```python
from build123d import *

# Parameters (mm, degrees)
F0_W     = 2.479451
F0_H     = 14.59062
F1_DEPTH = 2.54
F2_R     = 4.813733
F3_DEPTH = 1.27


with BuildPart() as f1:
    # F0 (on Top) → F1 (new body)
    with BuildSketch(Plane.XY):
        with Locations((-1.239726, -7.29531)):
            Rectangle(F0_W, F0_H)
    extrude(amount=F1_DEPTH)

    # F2 (on Front) → F3 (join)
    with BuildSketch(Plane.XZ):
        with Locations((-2.288725, 2.193361)):
            Circle(F2_R)
    extrude(amount=F3_DEPTH)


solid = f1.part
```
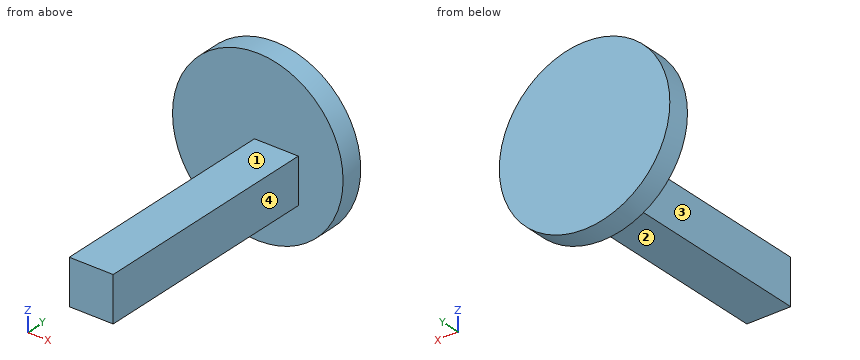
The listing builds one solid part. Answer for the finished solid, in the listing's coordinates (mm). Face numbers are marked on the shaded views. A direction names the side the tool comes from. Give positions to 0.01 mm unless a question says otherwise; leave off trailing zeros. Order: outer loops, then holes, each group sorted by start corner. A loop starts at its lowest first (then second) coordinate and runs counter-clockwise, first axis right, second up. Notation, with made-up numbers: (-34.75, -7.75) -> (-7.75, -7.75) arc R21 ccw to (-7.75, 30.25) -> close; hole circle Ø11 at (15, 58). An arc over 180 degrees is marked (long way). Answer as a JSON object with one key per item and string values. Group by question number.
Item 1: The part is cut by section D-D on z = -1. Write down the section's boundary in (x, y).
Item 2: The part is cut by section A-A on z = 0.75. Write down the section's boundary in (x, y).
Item 3: The part is cut by section B-B on x = -1.75. Write down the section's boundary in (y, z).
Item 4: Flat-ended cylindrical pins translate along their axes: pin 1 (0.8 mm diameter, centred on y = -8, z = 1, fed in from -X); pin 2 (0.7 mm diameter, centred on x = -1, y = -6, fed in from -Z); pin 3 (4 mm diameter, centred on x = 0.5, z = 5.5, fed in from -Y). Find the tip coordinate at first contact, or state that the pin passes through.
Item 5: A tool of negligible diameter and unlimited length cuts with its end or side. For the marked faces 1, 2, 3 and 4, from which of +Z, -Z, +X, -X, +Y, -Y can it reach the whole face along a straight path? Write none if from no direction.
Item 6: Consider L1, parallel to Y at x = -3, z = 0.25; L2, parallel to X at y = -5.5, z = 0.5; L3, parallel to Z at x = -2.25, y = -12.5. Determine where each line is inside the solid, lowest interval first. Write a range as from..to.
Item 7: The part is cut by section C-C on y = -10.25. Write down the section's boundary in (x, z).
Result set:
{
 "1": {"outline": "(-5.89, -1.27) -> (1.31, -1.27) -> (1.31, 0) -> (-5.89, 0) -> close"},
 "2": {"outline": "(-6.88, -1.27) -> (-2.48, -1.27) -> (-2.48, -14.59) -> (0, -14.59) -> (0, -1.27) -> (2.3, -1.27) -> (2.3, 0) -> (-6.88, 0) -> close"},
 "3": {"outline": "(-14.59, 0) -> (-1.27, 0) -> (-1.27, -2.59) -> (0, -2.59) -> (0, 6.98) -> (-1.27, 6.98) -> (-1.27, 2.54) -> (-14.59, 2.54) -> close"},
 "4": {"pin 1": "x = -2.48", "pin 2": "z = 0", "pin 3": "y = -1.27"},
 "5": {"face 1": "+Z, +X, -X, -Y", "face 2": "-Z, +X, -X, -Y", "face 3": "+Z, -Z, -X, -Y", "face 4": "+Z, -Z, +X, -Y"},
 "6": {"L1": "-1.27..0", "L2": "-2.48..0", "L3": "0..2.54"},
 "7": {"outline": "(-2.48, 0) -> (0, 0) -> (0, 2.54) -> (-2.48, 2.54) -> close"}
}
